Drawing for the job (mm, zero at the part's lowest x, y, z). A direction names the side the tool comes from. Round coordinates to 2 decimals unless told otherwise and drop trailing zeros. Order: outer loops, then holes, each group sorted by start corner. A loop starts at its lowest first (then second) coordinate and runs counter-clockwise, first axis right, second up. Notation, with made-up numbers: (3, -1.5) - (42, -1.5) arc R20 ccw to (42, 4.5) - close; hole circle Ø6 at (-27.75, 42). An arc over 180 degrees is marked (long way). Answer as a JSON object with one key per item and string values.
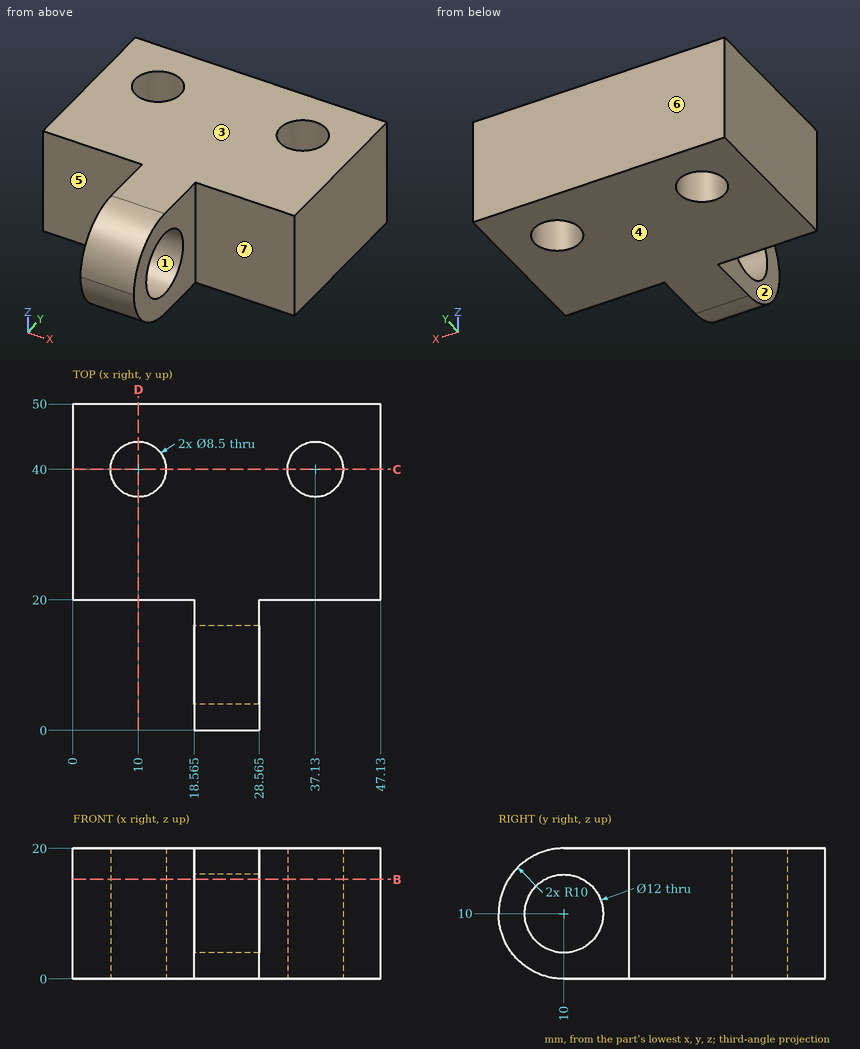
Item 1: Cut at B-B (z = 15.25). State how many separate pieces and enclosed holes the cut face has, plus the area to 3 significant figures.
Taken from the geometry:
{"separate pieces": "2", "enclosed holes": "2", "area": "1,430 mm2"}
Item 2: Cut at C-C (y = 40). Write the cut outline in (x, z).
Taken from the geometry:
{"outline": "(0, 0) - (5.75, 0) - (5.75, 20) - (0, 20) - close; (14.25, 0) - (32.88, 0) - (32.88, 20) - (14.25, 20) - close; (41.38, 0) - (47.13, 0) - (47.13, 20) - (41.38, 20) - close"}
Item 3: Two-plate mould, pull along Z, no slides. Class the marked faces 1, 2, 3 and 4: pulls with the +Z half, pulls with the -Z half, needs draft (parallel to the pull), parting line crosses it, or undercut.
Taken from the geometry:
{"face 1": "undercut", "face 2": "needs draft", "face 3": "pulls with the +Z half", "face 4": "pulls with the -Z half"}
Item 4: Tool access for the marked faces 5, 6 and 7: list every direction of +Z, -Z, +X, -X, +Y, -Y with a clear straight run to the whole face (end or side of a thin tool).
Taken from the geometry:
{"face 5": "+Z, -Z, -X, -Y", "face 6": "+Z, -Z, +X, -X, +Y", "face 7": "+Z, -Z, +X, -Y"}
Item 5: Cut at D-D (x = 10). Write the cut outline in (y, z), plus the area to 3 significant figures.
Taken from the geometry:
{"outline": "(20, 0) - (35.75, 0) - (35.75, 20) - (20, 20) - close; (44.25, 0) - (50, 0) - (50, 20) - (44.25, 20) - close", "area": "430 mm2"}
Item 6: Drop flat-ended pins along their axis: P1, Ø6, axis at y = 13.5, z = 5, coming from the -X side (3 decimals); P2, Ø5, axis at x = 23, z = 13.5, coming from the -Y side; P3, Ø4, axis at x = 34, z = 7, coming from the -Y side. Give the stop position or say it passes through.
Taken from the geometry:
{"P1": "x = 18.565", "P2": "y = 0.05", "P3": "y = 20"}
Item 7: Probe L1, parallel to Y at x = 22, z = 10; L2, parallel to Y at x = 10, z = 10.75; L3, parallel to Y at x = 3, z = 16. List the from-to ranges inside material, lowest first. Write a range as from..to.
Taken from the geometry:
{"L1": "0..4, 16..50", "L2": "20..35.75, 44.25..50", "L3": "20..50"}
